from build123d import *

# Parameters (mm, degrees)
SKETCH1_W                                        = 215.9
SKETCH1_H                                        = 50.8
BOSS_EXTRUDE1_DEPTH                              = 9.525
CSK_FOR_1_4_FLAT_HEAD_MACHINE_SCREW1_D           = 6.7564
CSK_FOR_1_4_FLAT_HEAD_MACHINE_SCREW1_CSINK_D     = 12.8778
CSK_FOR_1_4_FLAT_HEAD_MACHINE_SCREW1_CSINK_ANGLE = 82
F_5_16_18_TAPPED_HOLE1_D                         = 6.5278
F_5_16_18_TAPPED_HOLE1_CSINK_D                   = 9.2075
F_5_16_18_TAPPED_HOLE1_CSINK_ANGLE               = 82


with BuildPart() as part:
    # Sketch1 → Boss-Extrude1 (new body)
    with BuildSketch(Plane.XY):
        Rectangle(SKETCH1_W, SKETCH1_H)
    extrude(amount=BOSS_EXTRUDE1_DEPTH)

    # CSK for 1/4 Flat Head Machine Screw1 (through all)
    with Locations(Plane(origin=(0, 0, 0), x_dir=(-1, 0, 0), z_dir=(0, 0, -1))):
        with Locations((-95.25, 12.7), (-95.25, -12.7), (95.25, 12.7), (95.25, -12.7)):
            CounterSinkHole(CSK_FOR_1_4_FLAT_HEAD_MACHINE_SCREW1_D / 2, CSK_FOR_1_4_FLAT_HEAD_MACHINE_SCREW1_CSINK_D / 2, counter_sink_angle=CSK_FOR_1_4_FLAT_HEAD_MACHINE_SCREW1_CSINK_ANGLE)

    # 5/16-18 Tapped Hole1 (through all)
    with Locations(Plane.XY.offset(9.525)):
        with Locations((0, 0)):
            CounterSinkHole(F_5_16_18_TAPPED_HOLE1_D / 2, F_5_16_18_TAPPED_HOLE1_CSINK_D / 2, counter_sink_angle=F_5_16_18_TAPPED_HOLE1_CSINK_ANGLE)


solid = part.part
Verification items for the finished model (mm, model axes). Round coordinates to 2 decimals unless told otherwise and drop trailing zeros. Loops run counter-clockwise (first coordinate to the right, second up) from the corner with the lowest first, then second, coordinate; pieces in that order, holes last. Notation, with made-up numbers: (41, 88.5) - (55, 88.5) arc R17 ccw to (55, 113.5) - close; hole circle Ø1 at (24.25, 18.25). An arc over 180 degrees is marked (long way). Answer in a Markdown table with one row per item. Add a question column.
Q1. Material ranges on line 1 (Y direction, x = 95.25, z = 8.25); line 2 (X direction, y = -13, z = 9); line 3 (X direction, y = 15.5, z = 7.5), recorded low to high.
Q2. Gauge pin test, flat ends, axial feed: pin 1 (4 mm diameter, centred on x = 65.5, y = -19.5, fed in from -Z); pin 2 (4 mm diameter, centred on x = 0, y = 0, fed in from -Z); pin 3 (8 mm diameter, centred on x = -95.25, y = 12.7, fed in from -Z). Record the tip position at first contact, or that the pin passes through.
Q3. Section check B-B on y = -12.7. Enter the section's corners in (x, z) (3 decimals), plus the area to 3 significant figures.
Q4. Section check C-C on x = -95.25. Enter the section's corners in (y, z) (3 decimals).
Q5. Release check for a two-part mould opening along Y. For faces 1 (the face through (-91.99, 11.35, 3.35)), 2 (the face through (-2, -25.4, 5)), 3 (the face through (98.51, 11.35, 3.35)), 4 (the face through (-2, -5, 9.525)) record: pulls with the +Y half, pulls with the -Y half, needs draft (parallel to the pull), parting line crosses it, or undercut.
Q6. Section check A-A on x = 0. Enter the section's corners in (y, z) (3 decimals), plus the area to 3 significant figures.
Q7. Section check D-D on z = 1.5. Enter the section's corners in (x, y).
Found:
| question | item | result |
|---|---|---|
| 1 | line 1 | y = -25.4 to -16.08, -9.32 to 9.32, 16.08 to 25.4 |
| 1 | line 2 | x = -107.95 to -98.61, -91.89 to 91.89, 98.61 to 107.95 |
| 1 | line 3 | x = -107.95 to -97.14, -93.36 to 93.36, 97.14 to 107.95 |
| 2 | pin 1 | stops at z = 0 |
| 2 | pin 2 | passes through |
| 2 | pin 3 | stops at z = 2.81 |
| 3 | outline | (-107.95, 0) - (-101.689, 0) - (-98.628, 3.521) - (-98.628, 9.525) - (-107.95, 9.525) - close; (-91.872, 3.521) - (-88.811, 0) - (88.811, 0) - (91.872, 3.521) - (91.872, 9.525) - (-91.872, 9.525) - close; (98.628, 3.521) - (101.689, 0) - (107.95, 0) - (107.95, 9.525) - (98.628, 9.525) - close |
| 3 | area | 1,910 mm² |
| 4 | outline | (-25.4, 0) - (-19.139, 0) - (-16.078, 3.521) - (-16.078, 9.525) - (-25.4, 9.525) - close; (-9.322, 3.521) - (-6.261, 0) - (6.261, 0) - (9.322, 3.521) - (9.322, 9.525) - (-9.322, 9.525) - close; (16.078, 3.521) - (19.139, 0) - (25.4, 0) - (25.4, 9.525) - (16.078, 9.525) - close |
| 5 | face 1 | undercut |
| 5 | face 2 | pulls with the -Y half |
| 5 | face 3 | undercut |
| 5 | face 4 | needs draft |
| 6 | outline | (-25.4, 0) - (-3.264, 0) - (-3.264, 7.984) - (-4.604, 9.525) - (-25.4, 9.525) - close; (3.264, 0) - (25.4, 0) - (25.4, 9.525) - (4.604, 9.525) - (3.264, 7.984) - close |
| 6 | area | 420 mm² |
| 7 | outline | (-107.95, -25.4) - (107.95, -25.4) - (107.95, 25.4) - (-107.95, 25.4) - close; hole circle Ø10.27 at (-95.25, -12.7); hole circle Ø10.27 at (-95.25, 12.7); hole circle Ø6.53 at (0, 0); hole circle Ø10.27 at (95.25, -12.7); hole circle Ø10.27 at (95.25, 12.7) |
